For this review, take the finished solid that the model builds, in its own axes (mm). A direction names the side the tool comes from. Give positions to 0.01 mm unless a question says otherwise; leave off trailing zeros. Order: outer loops, then holes, each group sorted by start corner. A loop starts at its lowest first (then second) coordinate and runs counter-clockwise, first axis right, second up.
from build123d import *

# Parameters (mm, degrees)
F0_W     = 101.6
F0_H     = 94.322458
F1_DEPTH = 5
F0_H_2   = 4.017089
F0_H_3   = 3.260453
F2_DEPTH = 3


with BuildPart() as f1:
    # F0 (on Top) → F1 (new body)
    with BuildSketch(Plane.XY):
        Polygon((-50.8, -47.539547), (-50.8, 46.782911), (-71.69123, 28.25832), (-72.031133, -30.204607), align=None)
        with Locations((0, -0.378318)):
            Rectangle(F0_W, F0_H)
        Polygon((73.786288, 24.689363), (50.8, 46.782911), (50.8, -47.539547), (73.786288, -35.133168), align=None)
    extrude(amount=F1_DEPTH)

    # F0 (on Top) → F2 (join)
    with BuildSketch(Plane.XY):
        Polygon((-50.8, 46.782911), (-50.8, 50.8), (-74.547097, 29.664359), (-74.547097, -31.410809), (-50.8, -50.8), (-50.8, -47.539547), (-72.031133, -30.204607), (-71.69123, 28.25832), align=None)
        with Locations((0, 48.791455)):
            Rectangle(F0_W, F0_H_2)
        Polygon((76.217584, 26.386153), (50.8, 50.8), (50.8, 46.782911), (73.786288, 24.689363), (73.786288, -35.133168), (50.8, -47.539547), (50.8, -50.8), (76.217584, -37.332729), align=None)
        with Locations((0, -49.169773)):
            Rectangle(F0_W, F0_H_3)
    extrude(amount=F2_DEPTH)


solid = f1.part
1) Tool access review of faces 1 (the face through (62.454, 35.581, 3.986)), 2 (the face through (62.132, -41.423, 3.986)), 3 (the face through (-61.564, -38.751, 3.986)), 4 (the face through (-61.1, 37.65, 3.99)): name each direction out of +Z, -Z, +X, -X, +Y, -Y from which nothing blocks a thin tool from reaching the whole face with its end or side.
Answer sheet:
face 1: +Z, +X, +Y
face 2: +Z, +X, -Y
face 3: +Z, -X, -Y
face 4: +Z, -X, +Y
2) To check wall thickness, follow line 1 (Y direction, x = 25, z = 3.75); line 2 (X direction, y = 43, z = 3.6); line 3 (Y direction, x = 69.5, z = 4.85). State the ranges of each line that lie inside material, in increasing order.
Answer sheet:
line 1: y = -47.54 to 46.78
line 2: x = -55.07 to 54.74
line 3: y = -37.45 to 28.81
3) We need section A-A on z = 0.95. Give the boundary of the cut face in (x, y), then the cut area to 3 significant figures.
Answer sheet:
outline: (-74.55, -31.41) - (-50.8, -50.8) - (50.8, -50.8) - (76.22, -37.33) - (76.22, 26.39) - (50.8, 50.8) - (-50.8, 50.8) - (-74.55, 29.66) - close
area: 14,400 mm2
4) Clearance check with a flat-ended pin moving along its axis: pin 1 (0.6 mm diameter, centred on y = -4.5, z = 4, fed in from +X). State where the tip first meets the part, or that it passes through.
Answer sheet:
pin 1: stops at x = 73.79
5) We need section B-B on x = 42. Give the boundary of the cut face in (y, z), then the cut area to 3 significant figures.
Answer sheet:
outline: (-50.8, 0) - (50.8, 0) - (50.8, 3) - (46.78, 3) - (46.78, 5) - (-47.54, 5) - (-47.54, 3) - (-50.8, 3) - close
area: 493 mm2
